Check sheet for the modelled part. Datum: model origin and axes. Units: mm. Round coordinates to 2 decimals unless told otherwise and drop trailing zeros. Write each loop counter-clockwise with the first axis right and the second up, starting at its lowest first coordinate (ties: lowest second). Pieces come first, ordered by that corner, then holes.
from build123d import *

# Parameters (mm, degrees)
SKETCH1_R           = 17.46
SKETCH1_R_2         = 15
BOSS_EXTRUDE1_DEPTH = 1828.8
SKETCH4_W           = 2.08
SKETCH4_H           = 50
CUT_EXTRUDE2_DEPTH  = 141
SKETCH7_W           = 2.08
SKETCH7_H           = 50
CUT_EXTRUDE3_DEPTH  = 141


with BuildPart() as part:
    # Sketch1 → Boss-Extrude1 (new body)
    with BuildSketch(Plane.XY):
        Circle(SKETCH1_R)
        Circle(SKETCH1_R_2, mode=Mode.SUBTRACT)
    extrude(amount=BOSS_EXTRUDE1_DEPTH)

    # Sketch4 → Cut-Extrude2 (cut)
    with BuildSketch(Plane.XY):
        Rectangle(SKETCH4_W, SKETCH4_H)
    extrude(amount=CUT_EXTRUDE2_DEPTH, mode=Mode.SUBTRACT)

    # Sketch7 → Cut-Extrude3 (cut)
    with BuildSketch(Plane.XY.offset(1828.8)):
        Rectangle(SKETCH7_W, SKETCH7_H)
    extrude(amount=-CUT_EXTRUDE3_DEPTH, mode=Mode.SUBTRACT)


solid = part.part
1. Release check for a two-part mould opening along X. For faces 1 (the cylindrical face through (-14.985, 0.66, 901.598)), 2 (the cylindrical face through (-12.87, 11.8, 901.6)) record: released by +X, released by -X, zero draft, split by the parting line, or undercut.
2. Sectioned sample at B-B, the plane z = 1552.5. Enter the section's corners in (x, y), plus the area to 3 significant figures.
3. Scan lines: line 1 along X through (y, z) = (0, 1242.5); line 2 along Y through (x, z) = (1, 776.5); line 3 along X through (y, z) = (-2.5, 456.5). Record each from-to range of solid material in increasing order.
4. Go/stop test with flat-tipped pins: pin 1 (2 mm diameter, centred on y = 17, z = 65.5, fed in from -X); pin 2 (4 mm diameter, centred on x = 12, y = 11, fed in from -Z); pin 3 (2.5 mm diameter, centred on y = -16, z = 62, fed in from -X); pin 4 (1.2 mm diameter, centred on y = -15.5, z = 1768.5, fed in from -X). Record where each tip stops, or that it passes through.
5. Sectioned sample at C-C, the plane x = 9. Enter the section's corners in (y, z), plus the area to 3 significant figures.
6. Sectioned sample at A-A, the plane y = 0. Enter the section's corners in (x, z).
Computed values:
1. face 1: undercut
1. face 2: split by the parting line
2. outline: circle Ø34.92 at (0, 0); hole circle Ø30 at (0, 0)
2. area: 251 mm2
3. line 1: x = -17.46 to -15, 15 to 17.46
3. line 2: y = -17.43 to -14.97, 14.97 to 17.43
3. line 3: x = -17.28 to -14.79, 14.79 to 17.28
4. pin 1: stops at x = -6.99
4. pin 2: stops at z = 0
4. pin 3: stops at x = -9.34
4. pin 4: stops at x = -9.1
5. outline: (-14.96, 0) - (-12, 0) - (-12, 1828.8) - (-14.96, 1828.8) - close; (12, 0) - (14.96, 0) - (14.96, 1828.8) - (12, 1828.8) - close
5. area: 10,800 mm2
6. outline: (-17.46, 0) - (-15, 0) - (-15, 1828.8) - (-17.46, 1828.8) - close; (15, 0) - (17.46, 0) - (17.46, 1828.8) - (15, 1828.8) - close
